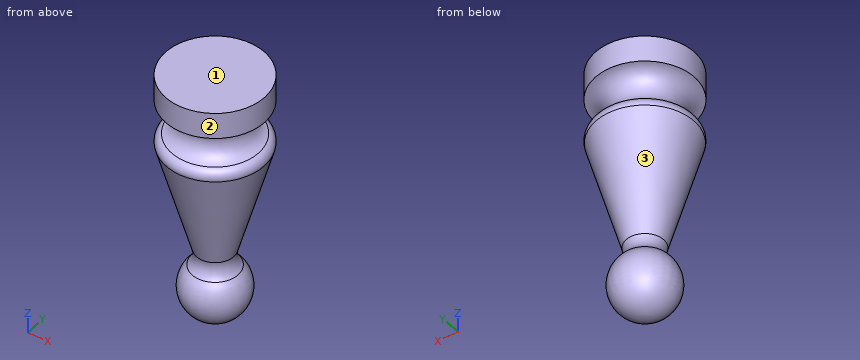
from build123d import *


with BuildPart() as part:
    # Sketch → Revolution (revolve)
    with BuildSketch(Plane.XZ):
        with BuildLine():
            Line((0, 0), (0, -28))
            ThreePointArc((0, -28), (3.213858, -25.886043), (2.545455, -22.09778))
            ThreePointArc((2.073267, -20.188708), (2.058505, -21.20529), (2.545455, -22.09778))
            Line((5.463367, -8.010997), (2.073267, -20.188708))
            ThreePointArc((5.463367, -8.010997), (5.387122, -7.281275), (4.833333, -6.8))
            ThreePointArc((5.5, -2.914382), (3.528803, -4.576178), (4.833333, -6.8))
            Line((5.5, -2.914382), (5.5, 0))
            Line((5.5, 0), (0, 0))
        make_face()
    revolve(axis=Axis((0, 0, 0), (0, 0, 1)))


solid = part.part
For this review, take the finished solid that the model builds, in its own axes (mm). Face numbers are marked on the shaded views. Coordinates: 2 decimals unless noted, no trailing zeros. Loops run counter-clockwise (first coordinate to the right, second up) from the corner with the lowest first, then second, coordinate; pieces in that order, holes last. Notation, with made-up numbers: (76.25, -20.75) - (90.25, -20.75) arc R14 ccw to (90.25, -3.75) - close; hole circle Ø2 at (33.25, 50). An arc over 180 degrees is marked (long way). Use a Markdown table: item, result. Add a question column.
Item 1: Insertion check: pin 1 Ø3 at (y, z) = (-1, -9) entering from +X; pin 2 Ø1.5 at (x, z) = (4, -12) entering from -Y; pin 3 Ø6 at (x, z) = (-3.5, -14.5) entering from +Y. Each pin has a flat end and moves straight along its axis. Give the tip position at first contact, or say it passes through.
Item 2: Mouldability with a two-part tool opening along Z and no side actions: class the marked faces 1, 2 and 3 as pulls with the +Z half, pulls with the -Z half, needs draft (parallel to the pull), parting line crosses it, or undercut.
Item 3: We need section A-A (z = -2.5). Give the boundary of the cut face in (x, y), and give its area (3 significant figures).
Item 4: For line 1 (X direction, y = 2.25, z = -8.5); line 2 (X direction, y = -0.75, z = -2.5); line 3 (Y direction, x = 0.5, z = -26.5), list the stretches that pass through material, from the lowest coordinate up.
Results list:
| question | item | result |
|---|---|---|
| 1 | pin 1 | stops at x = 5.5 |
| 1 | pin 2 | stops at y = -2.95 |
| 1 | pin 3 | stops at y = 4.02 |
| 2 | face 1 | pulls with the +Z half |
| 2 | face 2 | needs draft |
| 2 | face 3 | undercut |
| 3 | outline | circle Ø11 at (0, 0) |
| 3 | area | 95.0 mm^2 |
| 4 | line 1 | x = -4.83 to 4.83 |
| 4 | line 2 | x = -5.45 to 5.45 |
| 4 | line 3 | y = -2.83 to 2.83 |
